```python
from build123d import *

# Parameters (mm, degrees)
SKETCH1_R           = 1.1
BOSS_EXTRUDE1_DEPTH = 5


with BuildPart() as part:
    # Sketch1 → Boss-Extrude1 (new body)
    with BuildSketch(Plane.XY):
        with BuildLine():
            Line((-13.453363993, 84.941197291), (-12.514757203, 79.015067248))
            ThreePointArc((-12.514757203, 79.015067248), (0, 80), (12.514757203, 79.015067248))
            Line((12.514757203, 79.015067248), (13.453363993, 84.941197291))
            Line((13.453363993, 84.941197291), (14.079101854, 88.891950654))
            Line((14.079101854, 88.891950654), (15.017708644, 94.818080697))
            ThreePointArc((15.017708644, 94.818080697), (0, 96), (-15.017708644, 94.818080697))
            Line((-15.017708644, 94.818080697), (-14.079101854, 88.891950654))
            Line((-14.079101854, 88.891950654), (-13.453363993, 84.941197291))
        make_face()
        with Locations((-8, 88)):
            Circle(SKETCH1_R, mode=Mode.SUBTRACT)
        with Locations((8, 88)):
            Circle(SKETCH1_R, mode=Mode.SUBTRACT)
    extrude(amount=BOSS_EXTRUDE1_DEPTH)


solid = part.part
```
CAD build for the part. Positions are in the model's coordinates, mm. Round coordinates to 2 decimals unless told otherwise and drop trailing zeros. Write each loop counter-clockwise with the first axis right and the second up, starting at its lowest first coordinate (ties: lowest second). Pieces come first, ordered by that corner, then holes. Notation, with made-up numbers: (39, -29.5) -> (79, -29.5) arc R28 ccw to (79, -9.5) -> close; hole circle Ø3 at (-18, -28.5). An arc over 180 degrees is marked (long way). Answer in a Markdown table with one row per item. Add a question column.
Item 1: Saw through at B-B, the plane y = 88. Write the cut outline in (x, z), then the cut area to 3 significant figures.
Item 2: Saw through at A-A, the plane z = 0.55. Write the cut outline in (x, y).
Item 3: Saw through at D-D, the plane y = 82.25. Write the cut outline in (x, z), then the cut area to 3 significant figures.
Item 4: Saw through at C-C, the plane x = 8. Write the cut outline in (y, z), then the cut area to 3 significant figures.
Item 5: Mould opens along X. For faces 1 (the face through (8.59, 88.93, 2.46)), 2 (the face through (0, 96, 2)), 3 (the face through (0, 88, 0)), 4 (the face through (-7.41, 88.93, 2.46)) say: pulls with the +X half, pulls with the -X half, needs draft (parallel to the pull), parting line crosses it, or undercut.
Item 6: Drop flat-ended pins along their axis: pin 1 Ø2 at (x, z) = (-8.5, 3) entering from -Y; pin 2 Ø1.5 at (y, z) = (83, 1.5) entering from +X. Give the stop position or say it passes through.
Item 7: Drill centre lines: line 1 (X direction, y = 88, z = 1.9); line 2 (Y direction, x = -8, z = 2.3); line 3 (Y direction, x = -1, z = 3.5). Where is each one in solid material? Low to high. Write a range as from..to.
Findings below:
| question | item | result |
|---|---|---|
| 1 | outline | (-13.94, 0) -> (-9.1, 0) -> (-9.1, 5) -> (-13.94, 5) -> close; (-6.9, 0) -> (6.9, 0) -> (6.9, 5) -> (-6.9, 5) -> close; (9.1, 0) -> (13.94, 0) -> (13.94, 5) -> (9.1, 5) -> close |
| 1 | area | 117 mm^2 |
| 2 | outline | (-15.02, 94.82) -> (-12.51, 79.02) arc R80 cw to (12.51, 79.02) -> (15.02, 94.82) arc R96 ccw to start; hole circle Ø2.2 at (-8, 88); hole circle Ø2.2 at (8, 88) |
| 3 | outline | (-13.03, 0) -> (13.03, 0) -> (13.03, 5) -> (-13.03, 5) -> close |
| 3 | area | 130 mm^2 |
| 4 | outline | (79.6, 0) -> (86.9, 0) -> (86.9, 5) -> (79.6, 5) -> close; (89.1, 0) -> (95.67, 0) -> (95.67, 5) -> (89.1, 5) -> close |
| 4 | area | 69.3 mm^2 |
| 5 | face 1 | undercut |
| 5 | face 2 | parting line crosses it |
| 5 | face 3 | needs draft |
| 5 | face 4 | undercut |
| 6 | pin 1 | stops at y = 79.43 |
| 6 | pin 2 | stops at x = 13.26 |
| 7 | line 1 | x = -13.94..-9.1, -6.9..6.9, 9.1..13.94 |
| 7 | line 2 | y = 79.6..86.9, 89.1..95.67 |
| 7 | line 3 | y = 79.99..95.99 |
